Read the model definition and answer for the solid it produces. Units are mm, in the model's axes. Face numbers are marked on the shaded views. A direction names the side the tool comes from. Give positions to 0.01 mm unless a question says otherwise; leave off trailing zeros. Write each loop counter-clockwise with the first axis right and the second up, starting at its lowest first coordinate (ties: lowest second). Pieces come first, ordered by that corner, then holes. Notation, with made-up numbers: M -18,-14.5 L -7,-14.5 A13 ccw -7,8.5 Z; hole C 41,58.25 d7. An arc over 180 degrees is marked long. Use a Markdown table: item, result. Add a question column.
Item 1: For the marked faces 1, 2 and 3, determine the directions among +Z, -Z, +X, -X, +Y, -Y from which every point of the face is accessible in a straight line to the end or side of a thin tool.
Item 2: A cutting plane is placed at A-A on y = 1.55. Determine the outline of the cut face in (x, z).
Item 3: A cutting plane is placed at C-C on x = 12.5. Determine the outline of the cut face in (y, z), then the cut area to 3 significant figures.
Item 4: Consider probe 1 along Z at (x, y) = (18.5, 2.1); probe 2 along Z at (x, y) = (-15, 4.45); probe 3 along X at (y, z) = (1.6, 22.5). Determine where each line is inside the solid, lowest interval first. Write a range as [from, to].
Item 5: Given P1, Ø1.5, axis at y = 3, z = 23, coming from the -X side; P2, Ø2.5, axis at y = 3, z = -23, coming from the +X side; P3, Ø1, axis at x = 3.5, z = 4, coming from the -Y side; P4, Ø2.5, axis at y = 3, z = -21.5, coming from the -X side, each flat-ended and moving along its own axis, determine where each tip first touches the part or whether it passes through.
Item 6: A cutting plane is placed at B-B on x = 20.5. Determine the outline of the cut face in (y, z), then the cut area to 3 significant figures.
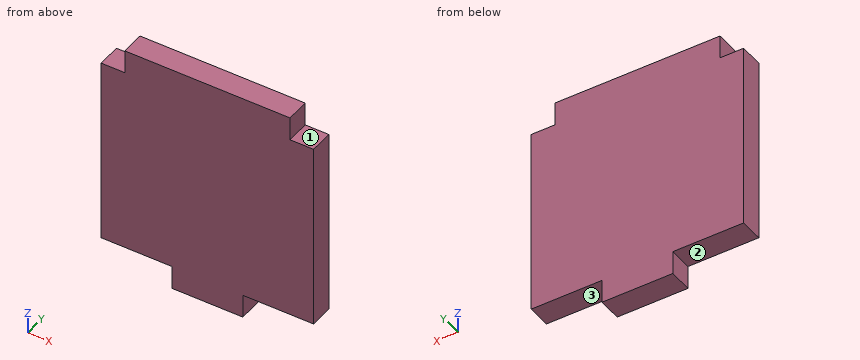
from build123d import *

# Parameters (mm, degrees)
SKETCH_1_W      = 45
SKETCH_1_H      = 40
SKETCH_1_W_2    = 35
SKETCH_1_H_2    = 5
EXTRUDE_1_DEPTH = 5
SKETCH_2_W      = 15
SKETCH_2_H      = 5
EXTRUDE_2_DEPTH = 5


with BuildPart() as part:
    # 草图1 → 凸台-拉伸1 (new body)
    with BuildSketch(Plane(origin=(0, 0, 0), x_dir=(1, 0, 0), z_dir=(0, 1, 0))):
        Rectangle(SKETCH_1_W, SKETCH_1_H)
        with Locations((0, -22.5)):
            Rectangle(SKETCH_1_W_2, SKETCH_1_H_2)
    extrude(amount=EXTRUDE_1_DEPTH)

    # 草图2 → 凸台-拉伸2 (add)
    with BuildSketch(Plane(origin=(0, 5, 0), x_dir=(1, 0, 0), z_dir=(0, 1, 0))):
        with Locations((0, 22.5)):
            Rectangle(SKETCH_2_W, SKETCH_2_H)
    extrude(amount=-EXTRUDE_2_DEPTH)


solid = part.part
Filled in:
| question | item | result |
|---|---|---|
| 1 | face 1 | +Z, +X, +Y, -Y |
| 1 | face 2 | -Z, -X, +Y, -Y |
| 1 | face 3 | -Z, +X, +Y, -Y |
| 2 | outline | M -22.5,-20 L -7.5,-20 L -7.5,-25 L 7.5,-25 L 7.5,-20 L 22.5,-20 L 22.5,20 L 17.5,20 L 17.5,25 L -17.5,25 L -17.5,20 L -22.5,20 Z |
| 3 | outline | M 0,-20 L 5,-20 L 5,25 L 0,25 Z |
| 3 | area | 225 mm² |
| 4 | probe 1 | [-20, 20] |
| 4 | probe 2 | [-20, 25] |
| 4 | probe 3 | [-17.5, 17.5] |
| 5 | P1 | x = -17.5 |
| 5 | P2 | x = 7.5 |
| 5 | P3 | y = 0 |
| 5 | P4 | x = -7.5 |
| 6 | outline | M 0,-20 L 5,-20 L 5,20 L 0,20 Z |
| 6 | area | 200 mm² |
